Here's how the part is built. I have some questions about the finished solid (model axes, mm). A direction names the side the tool comes from. Coordinates: 2 decimals unless noted, no trailing zeros. Order: outer loops, then holes, each group sorted by start corner. A loop starts at its lowest first (then second) coordinate and runs counter-clockwise, first axis right, second up. Notation, with made-up numbers: (55, -20) - (90, -20) arc R13 ccw to (90, 2) - close; hole circle Ø9 at (52, 26.5). An arc over 180 degrees is marked (long way). Use one line per item in the form item = value. Start each with the question number.
Autodesk Inventor part; units mm, degrees
ref_plane "Work Plane1" through (0, 12, 0) normal (0, 1, 0) x (1, 0, 0)
ref_plane "Work Plane2" through (0, 12, 0) normal (0, 1, 0) x (1, 0, 0)
ref_plane "YZ Plane" through (0, 0, 0) normal (1, 0, 0) x (0, 1, 0)
sketch "Sketch1" plane through (0, 0, 0) normal (0, 1, 0) x (-1, 0, 0)
  line L0 (-25, -43.3013) -> (-50, 0)
  line L1 (-50, 0) -> (-25, 43.3013)
  line L2 (-25, 43.3013) -> (25, 43.3013)
  line L3 (25, 43.3013) -> (50, 0)
  line L4 (50, 0) -> (25, -43.3013)
  line L5 (25, -43.3013) -> (-25, -43.3013)
  point P0 (0, 0)
  point P1 (0, 0)
  dimension "d0" = 50
extrude "Extrusion1" add sketch "Sketch1" along normal blind 12
ref_plane "Work Plane1" through (0, 12, 0) normal (0, 1, 0) x (1, 0, 0)
sketch "Sketch2" plane through (0, 12, 0) normal (0, 1, 0) x (1, 0, 0)
  circle A0 centre (0, 0) radius 17.5
  dimension "d4" = 35
extrude "Extrusion2" cut sketch "Sketch2" against normal blind 2
ref_plane "Work Plane2" through (0, 12, 0) normal (0, 1, 0) x (1, 0, 0)
sketch "Sketch3" plane through (0, 12, 0) normal (0, 1, 0) x (1, 0, 0)
  line L0 (-25, 43.3013) -> (-50, 0)
  line L1 (-50, 0) -> (-44, 0)
  circle A0 centre (-44, 0) radius 2.5
  line L2 (50, 0) -> (25, 43.3013)
  line L3 (25, 43.3013) -> (22, 38.1051)
  circle A1 centre (22, 38.1051) radius 2.5
  line L4 (25, -43.3013) -> (50, 0)
  line L5 (25, -43.3013) -> (22, -38.1051)
  circle A2 centre (22, -38.1051) radius 2.5
  point P0 (0, 0)
  dimension "d8" = 6
  dimension "d9" = 5
  dimension "d10" = 6
  dimension "d11" = 5
  dimension "d13" = 6
  dimension "d14" = 5
extrude "Extrusion3" cut sketch "Sketch3" against normal through all
properties part number "sensor 3"
1) Suppose I cut it at C-C, the plane z = -37. List the corners of the cut face in (x, y) for me.
2) I need wall thicknesses on probe 1 along Z at (x, y) = (22, 3.75); probe 2 along X at (y, z) = (9, 0); probe 3 along X at (y, z) = (6.5, -37). Which ranges of each line are inside material? Lowest first, please. Write a range as [from, to].
3) Which directions (+Z, -Z, +X, -X, +Y, -Y) give clear straight access to the entire face, cutting with the end or side of a thin tool? Please do faces 4 (the flat face through (37.3, 5.9, -22)), 5 (the flat face through (0, 10, 0)).
4) For pin 1 (2 mm diameter, centred on x = 7.5, z = -3.5, fed in from +Y); pin 2 (17.5 mm diameter, centred on x = -7.5, z = -6.5, fed in from +Y); pin 3 (2 mm diameter, centred on y = 6, z = -22, fed in from +X); pin 4 (1.5 mm diameter, centred on x = -30, y = 6, fed in from +Z), each with a flat end and sliding along its axis, tell me the tip position at first contact or that it passes through.
5) Suppose I cut it at B-B, the plane x = 0. List the corners of the cut face in (y, z) for me.
6) Suppose I cut it at A-A, the plane x = 22. List the corners of the cut face in (y, z) for me, then the cut area to 3 significant figures.
7) Suppose I cut it at D-D, the plane y = 5. List the corners of the cut face in (x, z) for me.
8) If we mould it in two halves opening along Z, with no side actions, what happens to faces 1 (the flat face through (0, 6, -43.301)), 2 (the cylindrical face through (-13.887, 11.014, 10.648)), 3 (the flat face through (1, 0, 1))? For each: pulls with the +Z half, pulls with the -Z half, needs draft (parallel to the pull), parting line crosses it, or undercut.
From the geometry:
q1.outline = (-28.64, 0) - (19.76, 0) - (19.76, 12) - (-28.64, 12) - close; (24.24, 0) - (28.64, 0) - (28.64, 12) - (24.24, 12) - close
q2.probe_1 = [-43.3, -40.61], [-35.61, 35.61], [40.61, 43.3]
q2.probe_2 = [-50, -46.5], [-41.5, 50]
q2.probe_3 = [-28.64, 19.76], [24.24, 28.64]
q3.face_4 = -Z, +X, +Y, -Y
q3.face_5 = +Y
q4.pin_1 = 10
q4.pin_2 = 12
q4.pin_3 = 37.88
q4.pin_4 = 35.94
q5.outline = (0, -43.3) - (12, -43.3) - (12, -17.5) - (10, -17.5) - (10, 17.5) - (12, 17.5) - (12, 43.3) - (0, 43.3) - close
q6.outline = (0, -43.3) - (12, -43.3) - (12, -40.61) - (0, -40.61) - close; (0, -35.61) - (12, -35.61) - (12, 35.61) - (0, 35.61) - close; (0, 40.61) - (12, 40.61) - (12, 43.3) - (0, 43.3) - close
q6.area = 919 mm2
q7.outline = (-50, 0) - (-25, -43.3) - (25, -43.3) - (50, 0) - (25, 43.3) - (-25, 43.3) - close; hole circle Ø5 at (-44, 0); hole circle Ø5 at (22, -38.11); hole circle Ø5 at (22, 38.11)
q8.face_1 = pulls with the -Z half
q8.face_2 = undercut
q8.face_3 = needs draft
